Read the model definition and answer for the solid it produces. Units are mm, in the model's axes. A direction names the side the tool comes from. Coordinates: 2 decimals unless noted, no trailing zeros. Loops run counter-clockwise (first coordinate to the right, second up) from the corner with the lowest first, then second, coordinate; pieces in that order, holes last. Notation, with made-up numbers: M 44.5,-30.75 L 77.5,-30.75 A19 cw 77.5,-21.75 Z; hole C 49.5,62 d11. An arc over 180 degrees is marked long. One line per item, written item: value. Start each with the question number.
```python
from build123d import *

# Parameters (mm, degrees)
SCHIZZO1_W                   = 15
SCHIZZO1_H                   = 70
ESTRUSIONE_ESTRUSIONE1_DEPTH = 5
SCHIZZO2_W                   = 5
SCHIZZO2_H                   = 15
ESTRUSIONE_ESTRUSIONE2_DEPTH = 3
SCHIZZO4_R                   = 1.5
TAGLIO_ESTRUSIONE2_DEPTH     = 6
SCHIZZO5_R                   = 0.25
TAGLIO_ESTRUSIONE3_DEPTH     = 10


with BuildPart() as part:
    # Schizzo1 → Estrusione-Estrusione1 (new body)
    with BuildSketch(Plane(origin=(0, 0, 0), x_dir=(0, 0, -1), z_dir=(1, 0, 0))):
        Rectangle(SCHIZZO1_W, SCHIZZO1_H)
    extrude(amount=ESTRUSIONE_ESTRUSIONE1_DEPTH)

    # Schizzo2 → Estrusione-Estrusione2 (add)
    with BuildSketch(Plane(origin=(0, 0, -7.5), x_dir=(-1, 0, 0), z_dir=(0, 0, -1))):
        with Locations((-2.5, 22.5)):
            Rectangle(SCHIZZO2_W, SCHIZZO2_H)
        with Locations((-2.5, -22.5)):
            Rectangle(SCHIZZO2_W, SCHIZZO2_H)
    extrude(amount=ESTRUSIONE_ESTRUSIONE2_DEPTH)

    # Schizzo4 → Taglio-Estrusione2 (cut, through all)
    with BuildSketch(Plane(origin=(0, 0, 0), x_dir=(0, 0, -1), z_dir=(1, 0, 0))):
        with Locations((2.5, 15)):
            Circle(SCHIZZO4_R)
        with Locations((2.5, -15)):
            Circle(SCHIZZO4_R)
        Polygon((-2.5, 1.25), (1.3, 1.25), (1.3, 2.75), (3.7, 2.75), (3.7, 1.25), (7.5, 1.25), (7.5, -1.25), (3.7, -1.25), (3.7, -2.75), (1.3, -2.75), (1.3, -1.25), (-2.5, -1.25), align=None)
    extrude(amount=TAGLIO_ESTRUSIONE2_DEPTH, mode=Mode.SUBTRACT)

    # Schizzo5 → Taglio-Estrusione3 (cut)
    with BuildSketch(Plane(origin=(5, 0, 0), x_dir=(0, 0, -1), z_dir=(1, 0, 0))):
        with Locations((3.7, 2.75)):
            Circle(SCHIZZO5_R)
        with Locations((3.7, -2.75)):
            Circle(SCHIZZO5_R)
    extrude(amount=-TAGLIO_ESTRUSIONE3_DEPTH, mode=Mode.SUBTRACT)


solid = part.part
```
1) For a pull along Z with two mould halves and no side action, classify faces 1 (the face through (2, 2, -3.7)), 2 (the face through (2, 0, 7.5)), 3 (the face through (0, 0, 3)) as released by +Z, released by -Z, zero draft, split by the parting line, or undercut.
2) A tool of negligible diameter and unlimited length cuts with its end or side. For faces 4 (the face through (3, -15, -9)), 5 (the face through (3, 30, -9)), 6 (the face through (2, -35, 0)), 7 (the face through (3, -30, -9)), 8 (the face through (2, -2, -1.3)), from which of +Z, -Z, +X, -X, +Y, -Y can it reach the whole face along a straight path? Write none if from no direction.
3) Section B-B (x = 1) is taken. Determine the outline of the cut face in (y, z).
4) Consider line 1 along Y through (x, z) = (2.4, -2.5); line 2 along Y through (x, z) = (1.4, 0.5); line 3 along Y through (x, z) = (2.7, -3). Determine where each line is inside the solid, lowest interval first.
5) Section A-A (z = 1.5) is taken. Determine the outline of the cut face in (x, y).
6) Section D-D (y = 5) is taken. Determine the outline of the cut face in (x, z), then the cut area to 3 significant figures.
7) Section C-C (z = -2.5) is taken. Determine the outline of the cut face in (x, y), then the cut area to 4 significant figures.
8) Flat-ended cylindrical pins translate along their axes: pin 1 (1.5 mm diameter, centred on x = 2.5, y = -33.5, fed in from -Z); pin 2 (2.5 mm diameter, centred on x = 1.5, z = -9.5, fed in from +Y). Find the tip coordinate at first contact, or state that the pin passes through.
Results found:
1. face 1: undercut
1. face 2: released by +Z
1. face 3: zero draft
2. face 4: -Z, +X, -X
2. face 5: -Z, +X, -X, +Y
2. face 6: +Z, -Z, +X, -X, -Y
2. face 7: -Z, +X, -X, -Y
2. face 8: +X, -X
3. outline: M -35,-7.5 L -30,-7.5 L -30,-10.5 L -15,-10.5 L -15,-7.5 L -1.25,-7.5 L -1.25,-3.7 L -2.5,-3.7 A0.25 cw long -2.75,-3.45 L -2.75,-1.3 L -1.25,-1.3 L -1.25,2.5 L 1.25,2.5 L 1.25,-1.3 L 2.75,-1.3 L 2.75,-3.45 A0.25 cw long 2.5,-3.7 L 1.25,-3.7 L 1.25,-7.5 L 15,-7.5 L 15,-10.5 L 30,-10.5 L 30,-7.5 L 35,-7.5 L 35,7.5 L -35,7.5 Z; hole C -15,-2.5 d3; hole C 15,-2.5 d3
4. line 1: y = -35 to -16.5, -13.5 to -2.75, 2.75 to 13.5, 16.5 to 35
4. line 2: y = -35 to -1.25, 1.25 to 35
4. line 3: y = -35 to -16.41, -13.59 to -2.75, 2.75 to 13.59, 16.41 to 35
5. outline: M 0,-35 L 5,-35 L 5,-1.25 L 0,-1.25 Z; M 0,1.25 L 5,1.25 L 5,35 L 0,35 Z
6. outline: M 0,-7.5 L 5,-7.5 L 5,7.5 L 0,7.5 Z
6. area: 75.0 mm²
7. outline: M 0,-35 L 5,-35 L 5,-16.5 L 0,-16.5 Z; M 0,-13.5 L 5,-13.5 L 5,-2.75 L 0,-2.75 Z; M 0,2.75 L 5,2.75 L 5,13.5 L 0,13.5 Z; M 0,16.5 L 5,16.5 L 5,35 L 0,35 Z
7. area: 292.5 mm²
8. pin 1: stops at z = -7.5
8. pin 2: stops at y = 30
